Geometry: final body of the model. Coordinates: model frame, mm. A direction names the side the tool comes from. Give positions to 0.01 mm unless a question says otherwise; leave off trailing zeros. Loops run counter-clockwise (first coordinate to the right, second up) from the corner with the lowest first, then second, coordinate; pieces in that order, holes last. Notation, with made-up numbers: M -2,-18.75 L 9,-18.75 A22 cw 9,13.25 Z; hole C -1,26 d3. An arc over 180 degrees is marked long. One line per question, with ' | ' between items. Start each with the question number.
from build123d import *

# Parameters (mm, degrees)
SKETCH2_W          = 55
SKETCH2_H          = 100
SKETCH3_R          = 50
CUT_EXTRUDE2_DEPTH = 95
SKETCH5_R          = 3
CUT_EXTRUDE4_DEPTH = 49


with BuildPart() as part:
    # Sketch2 → Revolve1 (revolve)
    with BuildSketch(Plane.XY, mode=Mode.PRIVATE) as revolve1_sk:
        with Locations((-10.224323353, 29.074307692)):
            Rectangle(SKETCH2_W, SKETCH2_H)
    revolve(revolve1_sk.sketch.rotate(Axis((17.275676647, -20.925692308, 0), (0, 1, 0)), 270), axis=Axis((17.275676647, -20.925692308, 0), (0, 1, 0)))

    # Sketch3 → Cut-Extrude2 (cut)
    with BuildSketch(Plane(origin=(0, 79.074307692, 0), x_dir=(1, 0, 0), z_dir=(0, 1, 0))):
        with Locations(Location((17.275676647, 0, 0), (0, 0, 270))):
            Circle(SKETCH3_R)
    extrude(amount=-CUT_EXTRUDE2_DEPTH, mode=Mode.SUBTRACT)

    # Sketch5 → Cut-Extrude4 (cut)
    with BuildSketch(Plane(origin=(75, 0, 0), x_dir=(0, 0, -1), z_dir=(1, 0, 0))):
        with Locations((0, 24.074307692)):
            Circle(SKETCH5_R)
    extrude(amount=-CUT_EXTRUDE4_DEPTH, mode=Mode.SUBTRACT)


solid = part.part
Q1. Section D-D, the plane y = 69. Output: boundary loops of the cut face in (x, z).
Q2. Contact query for flat-ended pins moving along their axis: pin 1 (3 mm diameter, centred on y = -10, z = 7, fed in from -X); pin 2 (3 mm diameter, centred on x = 28, z = 17, fed in from +Y); pin 3 (8 mm diameter, centred on x = -21.5, y = 11, fed in from +Z). Output: stop coordinate, or through.
Q3. Section A-A, the plane z = 0. Output: boundary loops of the cut face in (x, y), plus the area to 3 significant figures.
Q4. Set-up query: faces 4 (the flat face through (18, -15.926, -1)), 5 (the cylindrical face through (69.77, 27.05, 0.39)), 6 (the flat face through (17, -20.926, 1)). Return all of +Z, -Z, +X, -X, +Y, -Y with unobstructed straight access to the full face (end or side cutting, diameter ignored); none if empty.
Q5. Section C-C, the plane z = -26. Output: boundary loops of the cut face in (x, y), plus the area to 3 significant figures.
Q6. Material intervals for L1, parallel to Y at x = 69.25, z = 0; L2, parallel to X at y = 21, z = 0; L3, parallel to Z at x = 12, y = 13, sorted ascending.
Q7. Section B-B, the plane x = 59. Output: boundary loops of the cut face in (y, z).
Q8. Draft query along Z for faces 1 (the flat face through (66, 79.074, -12)), 2 (the cylindrical face through (38.341, 29.774, -50.806)), 3 (the cylindrical face through (32.294, 32.239, 47.691)). Return one class per face: released by +Z, released by -Z, zero draft, split by the parting line, or undercut.
Model answer:
1) outline: C 17.28,0 d110; hole C 17.28,0 d100
2) pin 1: stops at x = -37.45 | pin 2: stops at y = -15.93 | pin 3: stops at z = 42.61
3) outline: M -37.72,-20.93 L 72.28,-20.93 L 72.28,21.07 L 67.28,21.07 L 67.28,-15.93 L -32.72,-15.93 L -32.72,79.07 L -37.72,79.07 Z; M 67.28,27.07 L 72.28,27.07 L 72.28,79.07 L 67.28,79.07 Z | area: 1,470 mm^2
4) face 4: +Y | face 5: +X | face 6: +Z, -Z, +X, -X, -Y
5) outline: M -31.19,-20.93 L 65.74,-20.93 L 65.74,79.07 L 59.98,79.07 L 59.98,-15.93 L -25.43,-15.93 L -25.43,79.07 L -31.19,79.07 Z | area: 1,580 mm^2
6) L1: y = -20.93 to 21.07, 27.07 to 79.07 | L2: x = -37.72 to -32.72, 67.28 to 72.28 | L3: z = -54.75 to -49.72, 49.72 to 54.75
7) outline: M -20.93,-35.83 L 79.07,-35.83 L 79.07,-27.55 L -15.93,-27.55 L -15.93,27.55 L 79.07,27.55 L 79.07,35.83 L -20.93,35.83 Z
8) face 1: zero draft | face 2: split by the parting line | face 3: undercut
